```python
from build123d import *

# Parameters (mm, degrees)
F1_W     = 100
F1_H     = 100
F2_DEPTH = 5
F3_R     = 10
F5_D     = 9
F6_W     = 60
F6_H     = 5
F7_DEPTH = 50
F8_R     = 20
F10_D    = 26


# Not quite as in the source:
# - a pattern or mirror of a feature is missing from the dataset's text; its kind, count and spacing are read off the source's solid


with BuildPart() as f2:
    # F1 (on Top) → F2 (new body)
    with BuildSketch(Plane.XY):
        Rectangle(F1_W, F1_H)
    extrude(amount=F2_DEPTH)

    # F3
    f3_edges = [f2.edges().sort_by_distance(p)[0] for p in [
        (-50, 50, 2.5),
        (-50, -50, 2.5),
        (50, -50, 2.5),
        (50, 50, 2.5),
    ]]
    fillet(f3_edges, radius=F3_R)

    # F5 (through all)
    with Locations(Plane.XY.offset(5)):
        with Locations((-38, -38), (38, -38), (-38, -38), (38, 38)):
            f5 = Hole(F5_D / 2)

    # F5_copies: F5 across plane
    add(f5.mirror(Plane.ZX), mode=Mode.SUBTRACT)

    # F6 (on face) → F7 (join)
    with BuildSketch(Plane.XY.offset(5)):
        with Locations((0, -22.5)):
            Rectangle(F6_W, F6_H)
        with Locations((0, 22.5)):
            Rectangle(F6_W, F6_H)
    extrude(amount=F7_DEPTH)

    # F8
    f8_edges = [f2.edges().sort_by_distance(p)[0] for p in [
        (-30, -22.5, 55),
        (-30, 22.5, 55),
        (30, 22.5, 55),
        (30, -22.5, 55),
    ]]
    fillet(f8_edges, radius=F8_R)

    # F10 (through all)
    with Locations(Plane.XZ.offset(25)):
        with Locations((0, 30)):
            Hole(F10_D / 2)


solid = f2.part
```
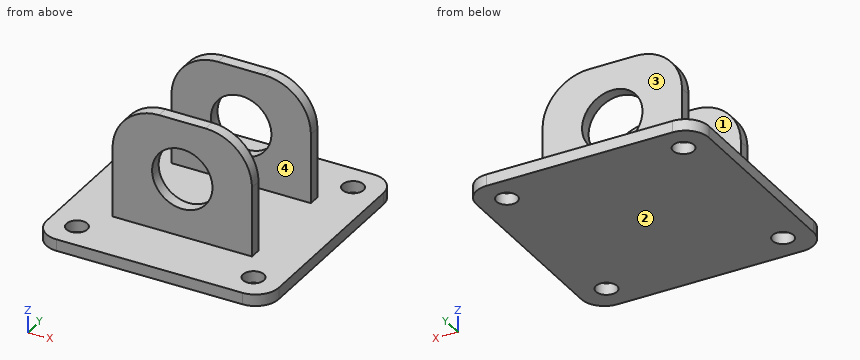
Geometry check sheet. Reference: the model listing, model coordinates, mm. Face numbers are marked on the shaded views. Round coordinates to 2 decimals unless told otherwise and drop trailing zeros. Loops run counter-clockwise (first coordinate to the right, second up) from the corner with the lowest first, then second, coordinate; pieces in that order, holes last. Notation, with made-up numbers: M 82.25,82.5 L 136.25,82.5 A22 ccw 136.25,107.5 Z; hole C 5,12.25 d1. An arc over 180 degrees is marked long. Return JSON: item names as keys, results as strings. Group by question number.
(1) Section check D-D, the plane z = 15. Enter the section's corners in (x, y).
(2) Section check A-A, the plane y = 38. Enter the section's corners in (x, z).
(3) Mould release check, pull along Y, two halves, no side actions. Record for the marked faces 1, 2, 3 and 4: pulls with the +Y half, pulls with the -Y half, needs draft (parallel to the pull), parting line crosses it, or undercut.
(4) Scan lines: line 1 along Y through (x, z) = (38, 3.6); line 2 along Y through (x, z) = (7.5, 13); line 3 along Z through (x, y) = (0, -21.85). Record each from-to range of solid material in increasing order. Write a range as [from, to].
(5) Go/stop test with flat-tipped pins: pin 1 (10.5 mm diameter, centred on x = 38, y = 38, fed in from +Z); pin 2 (4 mm diameter, centred on x = -6.5, z = 45, fed in from +Y); pin 3 (4 mm diameter, centred on x = -30, z = 36, fed in from -Y); pin 4 (23.5 mm diameter, centred on x = 0, z = 30, fed in from +Y). Record where each tip stops, or that it passes through.
(6) Section check C-C, the plane z = 30. Enter the section's corners in (x, y), and give its area (3 significant figures).
Data:
{
 "1": {"outline": "M -30,-25 L 30,-25 L 30,-20 L -30,-20 Z; M -30,20 L 30,20 L 30,25 L -30,25 Z"},
 "2": {"outline": "M -50,0 L -42.5,0 L -42.5,5 L -50,5 Z; M -33.5,0 L 33.5,0 L 33.5,5 L -33.5,5 Z; M 42.5,0 L 50,0 L 50,5 L 42.5,5 Z"},
 "3": {"face 1": "undercut", "face 2": "needs draft", "face 3": "pulls with the +Y half", "face 4": "undercut"},
 "4": {"line 1": "[-50, -42.5], [-33.5, 33.5], [42.5, 50]", "line 2": "[-25, -20], [20, 25]", "line 3": "[0, 17], [43, 55]"},
 "5": {"pin 1": "z = 5", "pin 2": "y = 25", "pin 3": "y = -25", "pin 4": "through"},
 "6": {"outline": "M -30,-25 L -13,-25 L -13,-20 L -30,-20 Z; M -30,20 L -13,20 L -13,25 L -30,25 Z; M 13,-25 L 30,-25 L 30,-20 L 13,-20 Z; M 13,20 L 30,20 L 30,25 L 13,25 Z", "area": "340 mm²"}
}
